Check sheet for the modelled part. Datum: model origin and axes. Units: mm. A direction names the side the tool comes from. Give positions to 0.01 mm unless a question says otherwise; leave off trailing zeros. Order: outer loops, then holes, each group sorted by start corner. A loop starts at its lowest first (then second) coordinate and runs counter-clockwise, first axis right, second up. Notation, with made-up numbers: M 14.5,-9.5 L 45.5,-9.5 A16 ccw 45.5,17.5 Z; hole C 5.5,19 d8. An arc over 180 degrees is marked long. Return JSON: item names as keys, results as strings. Group by question number.
from build123d import *

# Parameters (mm, degrees)
SKETCH2_W          = 3
SKETCH2_H          = 1
SKETCH3_R          = 1.55
CUT_EXTRUDE1_DEPTH = 13.369316877
CHAMFER1_SIZE      = 2


with BuildPart() as part:
    # Sketch2 → Revolve1 (revolve)
    with BuildSketch(Plane(origin=(0, 0, 0), x_dir=(1, 0, 0), z_dir=(0, 1, 0))):
        with Locations((1.5, -2.5)):
            Rectangle(SKETCH2_W, SKETCH2_H)
        with BuildLine():
            Line((0, 2), (0, -2))
            Line((0, -2), (3, -2))
            Line((3, -2), (3, -1))
            Line((3, -1), (4.267949192, -1))
            Line((4.267949192, -1), (6, -2))
            Line((6, -2), (8, -2))
            Line((8, -2), (8, -1))
            ThreePointArc((8, -1), (7, 0), (8, 1))
            Line((8, 1), (8, 2))
            Line((8, 2), (0, 2))
        make_face()
    revolve(axis=Axis((0, 0, 2), (0, 0, -1)))

    # Sketch3 → Cut-Extrude1 (cut, through all)
    with BuildSketch(Plane.XY.offset(3)):
        Circle(SKETCH3_R)
    extrude(amount=-CUT_EXTRUDE1_DEPTH, mode=Mode.SUBTRACT)

    # Chamfer1
    # the kernel refuses this chamfer: 2 mm, written as the material it adds along each edge
    with BuildSketch(Plane(origin=(0, 0, 1), x_dir=(1, 0, 0), z_dir=(0, 1, 0))) as chamfer1_piece_1_section:
        Polygon((3, -CHAMFER1_SIZE), (3 + CHAMFER1_SIZE, 0), (3, 0), align=None)
    chamfer1_piece_1 = revolve(axis=Axis((0, 0, 1), (0, 0, -1)), mode=Mode.PRIVATE)
    chamfer1_piece_1 = split(chamfer1_piece_1, bisect_by=Plane(origin=(-4.002141123, 0, 3), z_dir=(0, 0, -1)), keep=Keep.TOP, mode=Mode.PRIVATE)
    add(chamfer1_piece_1)


solid = part.part
1) Material ranges on line 1 along Z through (x, y) = (6.5, -4.5); line 2 along X through (y, z) = (3, 1.85); line 3 along Y through (x, z) = (0, 0.4), recorded low to high.
2) Sectioned sample at C-C on z = 1.75. Record the boundary of the cut face in (x, y), then the cut area to 3 significant figures.
3) Depth check by flat-ended pin: P1, Ø2.5, axis at x = 0, y = 0, coming from the -Z side; P2, Ø2, axis at x = 2, z = -1, coming from the +Y side; P3, Ø3, axis at x = 5, z = 2.5, coming from the -Y side. Enter the tip coordinate at first touch or a pass-through.
4) Sectioned sample at B-B on z = 0.8. Record the boundary of the cut face in (x, y).
5) Release check for a two-part mould opening along X. For faces 3 (the face through (0, 2, -2)), 4 (the face through (-1.73, 7.81, -1.51)), 5 (the face through (2.871, 1.191, 2.892)) record: released by +X, released by -X, zero draft, split by the parting line, or undercut.
6) Sectioned sample at D-D on z = -0.1. Record the boundary of the cut face in (x, y), then the cut area to 3 significant figures.
7) Sectioned sample at A-A on x = 0. Record the boundary of the cut face in (y, z), then the cut area to 3 significant figures.
8) Tool access check on faces 1 (the face through (-1.3, 1.3, 3)), 2 (the face through (2, -6, 2)). Record the directions out of +Z, -Z, +X, -X, +Y, -Y that give a thin tool (end or side, any length) a straight path to the whole face; none if there is none.
Reply:
{
 "1": {"line 1": "-2 to -1, 1 to 2", "line 2": "-7.42 to -4.89, -2.87 to 2.87, 4.89 to 7.42", "line 3": "-7.08 to -1.55, 1.55 to 7.08"},
 "2": {"outline": "C 0,0 d16; C 0,0 d8.5; hole C 0,0 d11.13; hole C 0,0 d3.1", "area": "153 mm^2"},
 "3": {"P1": "through", "P2": "y = 7.94", "P3": "y = -7.15"},
 "4": {"outline": "C 0,0 d14.8; hole C 0,0 d3.1"},
 "5": {"face 3": "zero draft", "face 4": "split by the parting line", "face 5": "undercut"},
 "6": {"outline": "C 0,0 d14.01; hole C 0,0 d3.1", "area": "147 mm^2"},
 "7": {"outline": "M -8,-2 L -1.55,-2 L -1.55,3 L -3,3 L -4.73,1.27 L -6,2 L -8,2 L -8,1 A1 cw -8,-1 Z; M 1.55,-2 L 8,-2 L 8,-1 A1 cw 8,1 L 8,2 L 6,2 L 4.73,1.27 L 3,3 L 1.55,3 Z", "area": "50.9 mm^2"},
 "8": {"face 1": "+Z, +X, -X, +Y, -Y", "face 2": "+Z"}
}
